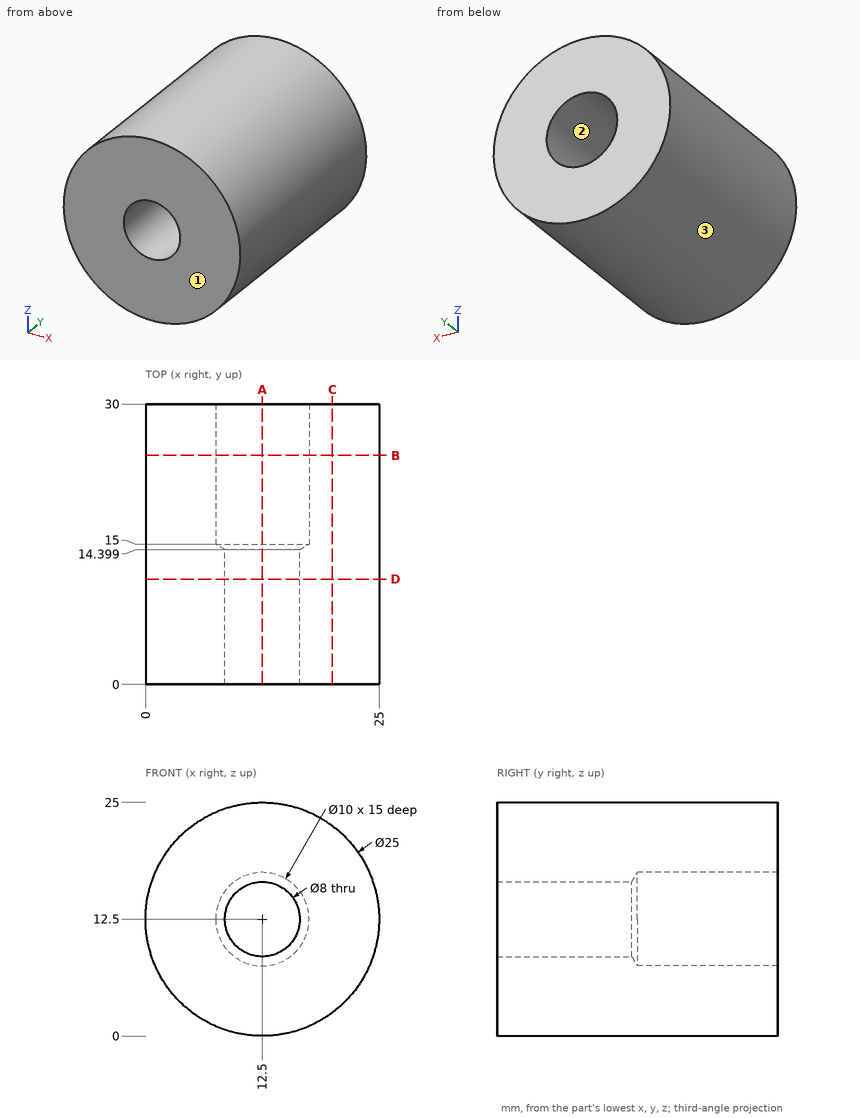
Design review of the part shown in the three views and the two pictorial views. Dimensions are in mm from the part's minimum x, y and z. Round coordinates to 2 decimals unless told otherwise and drop trailing zeros. Write each loop counter-clockwise with the first axis right and the second up, starting at its lowest first coordinate (ties: lowest second). Pieces come first, ordered by that corner, then holes.
Item 1: Draft analysis for pull direction X (two halves, no side actions). For the marked faces 1, 2 and 3, state which applies: released by +X, released by -X, zero draft, split by the parting line, or undercut.
Item 2: Consider section D-D on y = 11.25. Give the boundary of the cut face in (x, z), and give its area (3 significant figures).
Item 3: Consider section A-A on x = 12.5. Give the boundary of the cut face in (y, z).
Item 4: Consider section B-B on y = 24.5. Give the boundary of the cut face in (x, z).
Item 5: Consider section C-C on x = 20. Give the boundary of the cut face in (y, z), and give its area (3 significant figures).
Item 6: Wall thickness on L1, parallel to Z at x = 12.25, y = 28.75; L2, parallel to Z at x = 12, y = 6.75; L3, parallel to X at y = 25.5, z = 17: over which ranges is each line inside the solid? List them lowest first.
Item 7: For pin 1 Ø4 at (x, y) = (9.5, 7.5) entering from +Z; pin 2 Ø3 at (y, z) = (14, 8) entering from +X; pin 3 Ø1.5 at (x, y) = (11.5, 9.5) entering from -Z, all flat-tipped, find the tip position at first contact; note any pin that passes through.
Check values:
1. face 1: zero draft
1. face 2: undercut
1. face 3: split by the parting line
2. outline: circle Ø25 at (12.5, 12.5); hole circle Ø8 at (12.5, 12.5)
2. area: 441 mm2
3. outline: (0, 0) - (30, 0) - (30, 7.5) - (15, 7.5) - (14.4, 8.5) - (0, 8.5) - close; (0, 16.5) - (14.4, 16.5) - (15, 17.5) - (30, 17.5) - (30, 25) - (0, 25) - close
4. outline: circle Ø25 at (12.5, 12.5); hole circle Ø10 at (12.5, 12.5)
5. outline: (0, 2.5) - (30, 2.5) - (30, 22.5) - (0, 22.5) - close
5. area: 600 mm2
6. L1: z = 0 to 7.51, 17.49 to 25
6. L2: z = 0.01 to 8.53, 16.47 to 24.99
6. L3: x = 0.84 to 10.32, 14.68 to 24.16
7. pin 1: stops at z = 24.96
7. pin 2: stops at x = 24.63
7. pin 3: stops at z = 0
